Verification items for the finished model (mm, model axes). A direction names the side the tool comes from. Round coordinates to 2 decimals unless told otherwise and drop trailing zeros. Write each loop counter-clockwise with the first axis right and the second up, starting at its lowest first coordinate (ties: lowest second). Pieces come first, ordered by that corner, then holes. Notation, with made-up numbers: M 73,12 L 97,12 A30 cw 97,48 Z; hole C -1.75,-35 d2. An arc over 180 degrees is marked long. One line per question, with ' | ' between items. Start each with the question number.
Q1. Gauge pin test, flat end, axial feed: pin 1 (1.5 mm diameter, centred on x = 2, z = -30.5, fed in from +Y). Record the tip position at first contact, or that the pin passes through.
Q2. Release check for a two-part mould opening along Y. For faces 1 (the face through (1.48, -53.65, -0.07)), 2 (the face through (1.48, 10.1, 19.14)), 3 (the face through (1, -28, 20)) record: released by +Y, released by -Y, zero draft, split by the parting line, or undercut.
Q3. Tool access check on faces 4 (the face through (1.479, -0.215, -77.636)), 5 (the face through (1, -9, -32)). Record the directions out of +Z, -Z, +X, -X, +Y, -Y that give a thin tool (end or side, any length) a straight path to the whole face; none if there is none.
Q4. Thickness scan on line 1 along Y through (x, z) = (0.7, -76); line 2 along Y through (x, z) = (1.85, 15); line 3 along Z through (x, y) = (2.7, -53.5). Record the ranges inside material, lowest first. Write a range as from..to.
Q5. Cross-section at A-A (z = 0). Record the boundary of the cut face in (x, y).
Autodesk Inventor part; units mm, degrees
ref_plane "YZ Plane" through (0, 0, 0) normal (1, 0, 0) x (0, 1, 0)
ref_plane "XZ Plane" through (0, 0, 0) normal (0, 1, 0) x (-1, 0, 0)
ref_plane "XY Plane" through (0, 0, 0) normal (0, 0, 1) x (1, 0, 0)
sketch "Эскиз1" plane through (0, 0, 0) normal (1, 0, 0) x (0, 1, 0)
  circle A0 centre (0, 0) radius 1.65
  circle A1 centre (0, -76) radius 1.65
  circle A2 centre (-52, 0) radius 1.65
  circle A3 centre (-52, -76) radius 1.65
  line L0 (-63, 20) -> (8, 20)
  line L1 (8, -82) -> (-63, -82)
  line L2 (-66, -79) -> (-66, 17)
  arc A4 (11, 17) -> (8, 20) centre (8, 17) ccw
  arc A5 (8, -82) -> (11, -79) centre (8, -79) ccw
  arc A6 (-66, -79) -> (-63, -82) centre (-63, -79) ccw
  arc A7 (-63, 20) -> (-66, 17) centre (-63, 17) ccw
  circle A8 centre (-1.5, -43.6662) radius 1.65
  circle A9 centre (-50.5, -43.6662) radius 1.65
  circle A10 centre (-1.5, 14.3338) radius 1.65
  circle A11 centre (-50.5, 14.3338) radius 1.65
  line L3 (9, -39.8501) -> (-7, -39.8501)
  line L4 (-9, -37.8501) -> (-9, -26.8501)
  line L5 (-7, -24.8501) -> (9, -24.8501)
  line L6 (11, 17) -> (11, -22.8501)
  line L7 (11, -41.8501) -> (11, -79)
  arc A12 (-9, -37.8501) -> (-7, -39.8501) centre (-7, -37.8501) ccw
  arc A13 (-7, -24.8501) -> (-9, -26.8501) centre (-7, -26.8501) ccw
  arc A14 (9, -24.8501) -> (11, -22.8501) centre (9, -22.8501) ccw
  arc A15 (11, -41.8501) -> (9, -39.8501) centre (9, -41.8501) ccw
  point P0 (11, -39.8501)
  point P1 (-9, -39.8501)
  point P2 (-9, -24.8501)
  dimension "d4" = 3.3
  dimension "d8" = 3.3
  dimension "d13" = 3.3
  dimension "d14" = 3.3
  dimension "d20" = 3
  dimension "d23" = 52
  dimension "d29" = 3.3
  dimension "d31" = 3.3
  dimension "d34" = 3.3
  dimension "d35" = 3.3
  dimension "d36" = 20
  dimension "d37" = 15
  dimension "d38" = 2
extrude "Выдавливание2" add sketch "Эскиз1" along normal blind 3
properties part number "adapter_arduino_to_power"
Determined:
1) pin 1: stops at y = -9
2) face 1: undercut | face 2: released by +Y | face 3: zero draft
3) face 4: +X, -X | face 5: +X, -X, +Y
4) line 1: y = -66..-53.65, -50.35..-1.65, 1.65..11 | line 2: y = -66..-52.01, -48.99..-3.01, 0.01..11 | line 3: z = -82..-76.69, -75.31..-0.69, 0.69..20
5) outline: M 0,-66 L 3,-66 L 3,-53.65 L 0,-53.65 Z; M 0,-50.35 L 3,-50.35 L 3,-1.65 L 0,-1.65 Z; M 0,1.65 L 3,1.65 L 3,11 L 0,11 Z
